Could you check a few things on this model? Use its own coordinates, in mm. Face numbers are marked on the shaded views. A direction names the side the tool comes from. Round coordinates to 2 decimals unless told otherwise and drop trailing zeros. Loops run counter-clockwise (first coordinate to the right, second up) from the corner with the lowest first, then second, coordinate; pieces in that order, holes last. Notation, with made-up numbers: (70, 29) -> (77, 29) arc R23 ccw to (77, 38) -> close; hole circle Ø4 at (-12, -12.75). An arc over 180 degrees is marked (long way). Write each question's results on one line, items separated by ' | '.
from build123d import *

# Parameters (mm, degrees)
F1_DEPTH    = 100
F2_R        = 7
F3_T1_DEPTH = 386.6025403784
F4_T        = -3.2
F5_W        = 193.6
F5_H        = 20.7961232061
F6_DEPTH    = 4
F9_DEPTH    = 1.6
F10_W       = 61.8
F10_H       = 16.3858774256
F10_W_2     = 66.8
F11_DEPTH   = 3.25


# Not quite as in the source:
# - a fillet or chamfer that OpenCascade refuses, or shapes differently, is made with other operations: its cross-section is extruded or revolved along the edge and cut away or added
# - a pattern or mirror of a feature is missing from the dataset's text; its kind, count and spacing are read off the source's solid


with BuildPart() as f1:
    # F0 (on Right) → F1 (new body, symmetric)
    with BuildSketch(Plane.YZ):
        with BuildLine():
            ThreePointArc((-42.8978583449, -31.6602540378), (-46.8646250463, -29.7040611829), (-47.7274874763, -25.3661588123))
            Line((-47.7274874763, -25.3661588123), (-44.3324027769, -12.6955302183))
            Line((-44.3324027769, -12.6955302183), (-48.1961060821, -11.6602540378))
            Line((-48.1961060821, -11.6602540378), (-53.5550899307, -31.6602540378))
            Line((-53.5550899307, -31.6602540378), (-53.5550899307, -54.7542648054))
            Line((-53.5550899307, -54.7542648054), (57.1021416551, -54.7542648054))
            Line((57.1021416551, -54.7542648054), (-9.4337567297, -16.3397459622))
            Line((-9.4337567297, -16.3397459622), (9.4337567297, 16.3397459622))
            Line((9.4337567297, 16.3397459622), (5.9696551146, 18.3397459622))
            Line((5.9696551146, 18.3397459622), (-22.8978583449, -31.6602540378))
            Line((-22.8978583449, -31.6602540378), (-42.8978583449, -31.6602540378))
        make_face()
    extrude(amount=F1_DEPTH, both=True)

    # F2
    f2_edges = [f1.edges().sort_by_distance(p)[0] for p in [
        (0, -53.55509, -54.754265),
        (0, -9.433757, -16.339746),
        (0, -22.897858, -31.660254),
    ]]
    fillet(f2_edges, radius=F2_R)

    # F3: fillet of radius 10 on 1 edges, made by hand

    # F3_s2 → F3_t1 (cut)
    with BuildSketch(Plane.YZ.offset(-193.3012701892)):
        with BuildLine():
            ThreePointArc((24.7816335794, -36.0940107676), (29.4408918423, -47.3424552565), (19.7816335794, -54.7542648054))
            Line((19.7816335794, -54.7542648054), (57.1021416551, -54.7542648054))
            Line((57.1021416551, -54.7542648054), (24.7816335794, -36.0940107676))
        make_face()
    extrude(amount=F3_T1_DEPTH, mode=Mode.SUBTRACT)

    # F4 (hollow: no face is removed)
    offset(amount=F4_T, mode=Mode.SUBTRACT)

    # F5 (on face) → F6 (cut)
    with BuildSketch(Plane.XZ.offset(53.5550899307)):
        with Locations((0, -41.1562032024)):
            Rectangle(F5_W, F5_H)
    extrude(amount=-F6_DEPTH, mode=Mode.SUBTRACT)

    # F8 (on offset) → F9 (join)
    with BuildSketch(Plane.YZ.offset(35)):
        with BuildLine():
            Line((-49.5550899307, -31.4478701056), (-49.5550899307, -30.7581415993))
            Line((-49.5550899307, -30.7581415993), (-53.3133696313, -30.7581415993))
            Line((-53.3133696313, -30.7581415993), (-53.5550899307, -47.7542648054))
            ThreePointArc((-53.5550899307, -47.7542648054), (-53.2689348678, -49.735245916), (-52.4338653134, -51.5542648054))
            Line((-52.4338653134, -51.5542648054), (-46.5550899307, -51.5542648054))
            Line((-46.5550899307, -51.5542648054), (19.7816335794, -51.5542648054))
            ThreePointArc((19.7816335794, -51.5542648054), (26.3499291982, -46.5142343121), (23.1816335794, -38.8652920597))
            Line((23.1816335794, -38.8652920597), (-4.9715789032, -22.6110272543))
            ThreePointArc((-4.9715789032, -22.6110272543), (-8.2208411642, -19.6367335794), (-9.9129123978, -15.569667924))
            Line((-9.9129123978, -15.569667924), (-18.1058511106, -29.7602540378))
            ThreePointArc((-18.1058511106, -29.7602540378), (-21.8393102292, -33.4937131564), (-26.9393102292, -34.8602540378))
            Line((-26.9393102292, -34.8602540378), (-42.8978583449, -34.8602540378))
            ThreePointArc((-42.8978583449, -34.8602540378), (-46.6382826687, -33.9574607553), (-49.5550899307, -31.4478701056))
        make_face()
    f9 = extrude(amount=-F9_DEPTH)

    # F9_copies: F9 across plane
    add(f9.mirror(Plane(origin=(0, 0, 0), x_dir=(0, 0, -1), z_dir=(-1, 0, 0))))

    # F10 (on face) → F11 (cut)
    with BuildSketch(Plane(origin=(0, -3.4641016151, 2), x_dir=(1, 0, 0), z_dir=(0, -0.8660254038, 0.5))):
        with Locations((-65.9, -26.6331228623)):
            Rectangle(F10_W, F10_H)
        with Locations((0, -26.6331228623)):
            Rectangle(F10_W_2, F10_H)
        with Locations((65.9, -26.6331228623)):
            Rectangle(F10_W, F10_H)
    extrude(amount=-F11_DEPTH, mode=Mode.SUBTRACT)


solid = f1.part
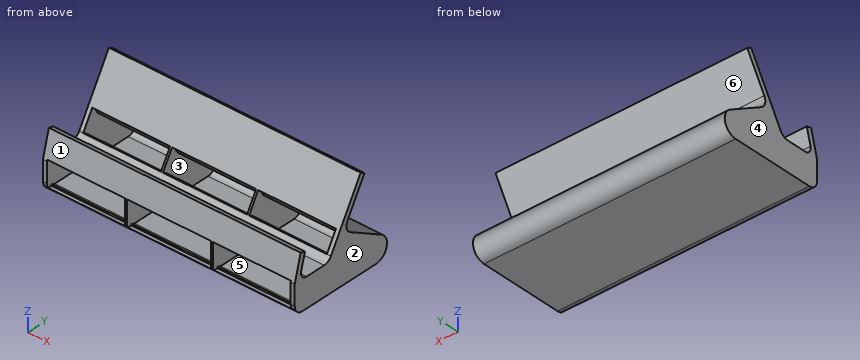
1) I want a section at C-C, the plane z = -44.5. Write out the boundary of the cut face in (x, y), plus the area to 3 significant figures.
Model answer:
outline: (-100, -53.56) -> (-96.8, -53.56) -> (-96.8, 26.58) -> (-35, 26.58) -> (-35, -53.51) -> (-33.4, -53.51) -> (-33.4, 26.58) -> (33.4, 26.58) -> (33.4, -53.51) -> (35, -53.51) -> (35, 26.58) -> (96.8, 26.58) -> (96.8, -53.56) -> (100, -53.56) -> (100, 29.78) -> (-100, 29.78) -> close | area: 1,410 mm2
2) I need wall thicknesses on line 1 (X direction, y = -15, z = -23); line 2 (Z direction, x = 69.5, y = -6); line 3 (Z direction, x = 3.5, y = -29.5). Which ranges of each line are inside material? Lowest first, please.
Model answer:
line 1: x = -100 to -96.8, -35 to -33.4, 33.4 to 35, 96.8 to 100 | line 2: z = -54.75 to -51.55, -21.93 to -17.16, -10.39 to -2.39 | line 3: z = -54.75 to -51.55, -34.86 to -31.66
3) If we mould it in two halves opening along Z, with no side actions, what happens to the marked faces 1, 2 and 3? For each: released by +Z, released by -Z, zero draft, split by the parting line, or undercut.
Model answer:
face 1: released by +Z | face 2: zero draft | face 3: undercut
4) I want a section at D-D, the plane z = -5. Write out the boundary of the cut face in (x, y), plus the area to 3 significant figures.
Model answer:
outline: (-100, -7.51) -> (100, -7.51) -> (100, -2.89) -> (-100, -2.89) -> close | area: 924 mm2
5) For the marked faces 4, 5 and 6, which set-ups out of +Z, -Z, +X, -X, +Y, -Y let a thin tool reach every point of the face, with its end or its side?
Model answer:
face 4: +Z, -Z, -X, +Y, -Y | face 5: none | face 6: +X, -X, +Y
6) I'm going to push flat-ended pins straight in: pin 1 (0.6 mm diameter, centred on x = -57, z = -31, fed in from -Y); pin 2 (12 mm diameter, centred on x = -66, z = 0.5, fed in from -Y); pin 3 (6 mm diameter, centred on x = 44, z = -34, fed in from -Y). Where does each tip first touch, or does it pass through?
Model answer:
pin 1: stops at y = -53.31 | pin 2: stops at y = -7.79 | pin 3: stops at y = -49.56
7) I want a section at B-B, the plane z = -18. Write out the boundary of the cut face in (x, y).
Model answer:
outline: (-100, -49.89) -> (100, -49.89) -> (100, -45.75) -> (-100, -45.75) -> close; (-100, -15.01) -> (-96.8, -15.01) -> (-96.8, -9.16) -> (-35, -9.16) -> (-35, -15.01) -> (-33.4, -15.01) -> (-33.4, -9.16) -> (33.4, -9.16) -> (33.4, -15.01) -> (35, -15.01) -> (35, -9.16) -> (96.8, -9.16) -> (96.8, -15.01) -> (100, -15.01) -> (100, -5.45) -> (-100, -5.45) -> close
